```python
from build123d import *

# Parameters (mm, degrees)
F1_DEPTH = 6.35
F3_R     = 6.34999
F4_D     = 6.9088


# Not quite as in the source:
# - a fillet or chamfer is up to 0.001 mm smaller than in the source, because OpenCascade refuses the exact size


with BuildPart() as f1:
    # F0 (on Front) → F1 (new body, symmetric)
    with BuildSketch(Plane.XZ):
        Polygon((0, 12.7), (0, 0), (101.6, 0), (101.6, 3.175), (68.3823774224, 12.7), align=None)
    extrude(amount=F1_DEPTH, both=True)

    # F3 (radius 6.35 in the source; OpenCascade refuses exactly that, so slightly less here)
    f3_edges = [f1.edges().sort_by_distance(p)[0] for p in [
        (0, -6.35, 6.35),
        (0, 6.35, 6.35),
    ]]
    fillet(f3_edges, radius=F3_R)

    # F4 (through all)
    with Locations(Plane.XY.offset(12.7)):
        with Locations((52.4002, 0), (7.9502, 0)):
            Hole(F4_D / 2)


solid = f1.part
```
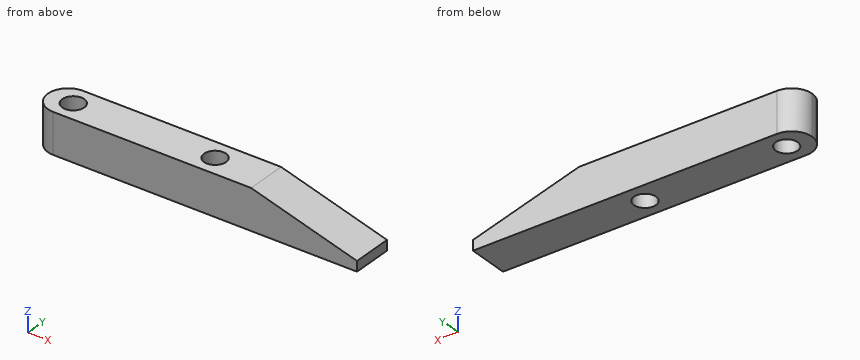
The listing builds one solid part. Answer for the finished solid, in the listing's coordinates (mm). Give positions to 0.01 mm unless a question says otherwise; leave off trailing zeros. Order: outer loops, then holes, each group sorted by start corner. A loop starts at its lowest first (then second) coordinate and runs counter-clockwise, first axis right, second up.
1) Find section C-C on x = 52.5. Write down the section's boundary in (y, z).
Reported:
outline: (-6.35, 0) - (-3.45, 0) - (-3.45, 12.7) - (-6.35, 12.7) - close; (3.45, 0) - (6.35, 0) - (6.35, 12.7) - (3.45, 12.7) - close
2) Find section A-A on y = 1.75. Write down the section's boundary in (x, z) (3 decimals), then the cut area to 3 significant figures.
Reported:
outline: (0.246, 0) - (4.972, 0) - (4.972, 12.7) - (0.246, 12.7) - close; (10.929, 0) - (49.422, 0) - (49.422, 12.7) - (10.929, 12.7) - close; (55.379, 0) - (101.6, 0) - (101.6, 3.175) - (68.382, 12.7) - (55.379, 12.7) - close
area: 978 mm2
3) Find section D-D on x = 90.5. Write down the section's boundary in (y, z), then the cut area to 3 significant figures.
Reported:
outline: (-6.35, 0) - (6.35, 0) - (6.35, 6.36) - (-6.35, 6.36) - close
area: 80.7 mm2
4) Given P1, Ø4, axis at x = 7.95, y = 0, coming from the +Z side; P2, Ø1.5, axis at y = -3, z = 4, coming from the -X side, each flat-ended and moving along its own axis, determine where each tip first touches the part or whether it passes through.
Reported:
P1: passes through
P2: stops at x = 0.41
5) Consider line 1 along Y through (x, z) = (51.5, 6.75); line 2 along Y through (x, z) = (8, 2); line 3 along Z through (x, y) = (97, 3.5). Determine where each line is inside the solid, lowest interval first.
Reported:
line 1: y = -6.35 to -3.34, 3.34 to 6.35
line 2: y = -6.35 to -3.45, 3.45 to 6.35
line 3: z = 0 to 4.49
6) Find section B-B on z = 10. Give the number of separate pieces and of enclosed holes in the cut face, then the cut area to 3 significant figures.
Reported:
separate pieces: 1
enclosed holes: 2
area: 896 mm2
